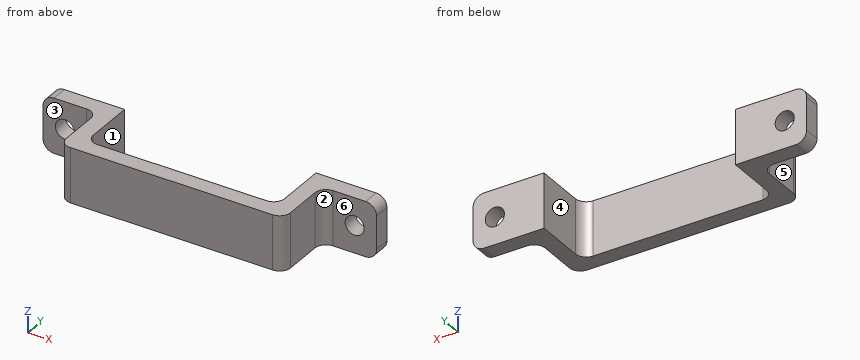
from build123d import *

# Parameters (mm, degrees)
EXTRUDE_THIN1_DEPTH = 5
FILLET1_R           = 2
FILLET2_R           = 2
SKETCH2_R           = 1.75
CUT_EXTRUDE1_DEPTH  = 4


with BuildPart() as part:
    # Sketch1 → Extrude-Thin1 (new body, symmetric)
    with BuildSketch(Plane.XY):
        Polygon((-30.5, 0), (-17.5, 0), (-17.5, -11), (17.5, -11), (17.5, 0), (30.5, 0), (30.5, -3), (20.5, -3), (20.5, -14), (-20.5, -14), (-20.5, -3), (-30.5, -3), align=None)
    extrude(amount=EXTRUDE_THIN1_DEPTH, both=True)

    # Fillet1
    fillet1_edges = [part.edges().sort_by_distance(p)[0] for p in [
        (20.5, -3, 0),
        (20.5, -14, 0),
        (-20.5, -14, 0),
        (-20.5, -3, 0),
        (-17.5, -11, 0),
        (17.5, -11, 0),
    ]]
    fillet(fillet1_edges, radius=FILLET1_R)

    # Fillet2
    fillet2_edges = [part.edges().sort_by_distance(p)[0] for p in [
        (-30.5, -1.5, -5),
        (30.5, -1.5, -5),
        (-30.5, -1.5, 5),
        (30.5, -1.5, 5),
    ]]
    fillet(fillet2_edges, radius=FILLET2_R)

    # Sketch2 → Cut-Extrude1 (cut, through all)
    with BuildSketch(Plane(origin=(0, -3, 0), x_dir=(-1, 0, 0), z_dir=(0, -1, 0))):
        with Locations((-26.5, 0)):
            Circle(SKETCH2_R)
        with Locations((26.5, 0)):
            Circle(SKETCH2_R)
    extrude(amount=-CUT_EXTRUDE1_DEPTH, mode=Mode.SUBTRACT)


solid = part.part
CAD build for the part. Positions are in the model's coordinates, mm. Face numbers are marked on the shaded views. A direction names the side the tool comes from. Round coordinates to 2 decimals unless told otherwise and drop trailing zeros. Order: outer loops, then holes, each group sorted by start corner. A loop starts at its lowest first (then second) coordinate and runs counter-clockwise, first axis right, second up. Notation, with made-up numbers: M 83.5,-33.75 L 101.5,-33.75 A12 cw 101.5,-10.75 Z; hole C -15.75,41 d8. An arc over 180 degrees is marked long. Use one line per item in the form item = value.
Q1. Saw through at C-C on x = 26.5. Give the cut face in (y, z).
Recorded:
outline = M -3,-5 L 0,-5 L 0,-1.75 L -3,-1.75 Z; M -3,1.75 L 0,1.75 L 0,5 L -3,5 Z
Q2. Saw through at D-D on z = 4. Give the cut face in (x, y), then the cut area to 3 significant figures.
Recorded:
outline = M -30.23,-3 L -22.5,-3 A2 cw -20.5,-5 L -20.5,-12 A2 ccw -18.5,-14 L 18.5,-14 A2 ccw 20.5,-12 L 20.5,-5 A2 cw 22.5,-3 L 30.23,-3 L 30.23,0 L 17.5,0 L 17.5,-9 A2 cw 15.5,-11 L -15.5,-11 A2 cw -17.5,-9 L -17.5,0 L -30.23,0 Z
area = 249 mm^2
Q3. Which spindle directions (+Z, -Z, +X, -X, +Y, -Y) get a long thin tool onto all of the face, cutting with end or side? Do the marked faces 4, 5 and 6. Say none if no direction does.
Recorded:
face_4 = +Z, -Z, +Y
face_5 = +Z, -Z, -X, -Y
face_6 = +Z, -Z, +X, -Y
Q4. Two-plate mould, pull along X, no slides. Class the marked faces 1, 2 and 3: +X half, -X half, draft (parallel to the pull), parting line (faces both ways), or undercut.
Recorded:
face_1 = undercut
face_2 = +X half
face_3 = draft
Q5. Probe L1, parallel to X at y = -1.4, z = 0; L2, parallel to X at y = -8.25, z = 3.75; L3, parallel to Z at x = -26.5, y = -1.55. List the from-to ranges inside material, lowest first.
Recorded:
L1 = -30.5 to -28.25, -24.75 to -17.5, 17.5 to 24.75, 28.25 to 30.5
L2 = -20.5 to -17.5, 17.5 to 20.5
L3 = -5 to -1.75, 1.75 to 5
Q6. Flat gauge pins, fed straight in: P1, Ø3.5, axis at y = -7, z = 1.5, coming from the -X side; P2, Ø3, axis at x = 6, z = 1, coming from the +Y side; P3, Ø3.5, axis at y = -8, z = 2.5, coming from the +X side. Where does each tip first touch, or does it go through?
Recorded:
P1 = -20.5
P2 = -11
P3 = 20.5
Q7. Saw through at B-B on z = 0. Give the cut face in (x, y).
Recorded:
outline = M -30.5,-3 L -28.25,-3 L -28.25,0 L -30.5,0 Z; M -24.75,-3 L -22.5,-3 A2 cw -20.5,-5 L -20.5,-12 A2 ccw -18.5,-14 L 18.5,-14 A2 ccw 20.5,-12 L 20.5,-5 A2 cw 22.5,-3 L 24.75,-3 L 24.75,0 L 17.5,0 L 17.5,-9 A2 cw 15.5,-11 L -15.5,-11 A2 cw -17.5,-9 L -17.5,0 L -24.75,0 Z; M 28.25,-3 L 30.5,-3 L 30.5,0 L 28.25,0 Z
Q8. Saw through at A-A on y = -8. Give the cut face in (x, z).
Recorded:
outline = M -20.5,-5 L -17.5,-5 L -17.5,5 L -20.5,5 Z; M 17.5,-5 L 20.5,-5 L 20.5,5 L 17.5,5 Z
